Input: part model. Units: mm. Frame: model coordinates. A direction names the side the tool comes from. Round coordinates to 2 decimals unless told otherwise and drop trailing zeros. Loops run counter-clockwise (first coordinate to the right, second up) from the corner with the lowest first, then second, coordinate; pieces in that order, holes last.
(1) Line query: line 1 (X direction, y = 7.25, z = 0); line 2 (Z direction, x = -8, y = 5.5); line 3 (Y direction, x = -20.5, z = -18). Output: solid intervals per line, ascending.
(2) First-contact query: pin 1 Ø0.8 at (y, z) = (4.5, 26) entering from +X; pin 2 Ø0.5 at (x, z) = (-2.5, 30) entering from -Y; pin 3 Ø20.5 at (y, z) = (-0.5, 44.5) entering from +X. Flat tips, straight axial feed; report the tip coordinate or a pass-through.
(3) Cut plane B-B, the plane x = 22. Output: boundary loops of the cut face in (y, z), and give its area (3 significant figures).
(4) Cut plane A-A, the plane z = 0. Output: boundary loops of the cut face in (x, y).
(5) Cut plane D-D, the plane y = -13. Output: boundary loops of the cut face in (x, z), and give its area (3 significant figures).
(6) Cut plane C-C, the plane y = 4. Output: boundary loops of the cut face in (x, z).
(7) Draft query along X for faces 1 (the face through (0, -20, 78)), 2 (the face through (-29.97, 4.93, -1.32)), 3 (the face through (-5, 0, 56)), 4 (the face through (-2.5, 5, -22)). Return one class per face: released by +X, released by -X, zero draft, split by the parting line, or undercut.
(8) Access query for faces 5 (the face through (24.995, 4.93, -0.515)), 6 (the face through (0.07, -2.89, 53.9)), 7 (the face through (0.81, -14.93, 84.31)), 8 (the face through (5, 0, 56)). Directions: +Z, -Z, +X, -X, +Y, -Y. A direction counts if a zero-diameter tool reaches every point of the face in a straight line with its end or side. Return the directions, or none.
from build123d import *

# Parameters (mm, degrees)
SKETCH1_R           = 30
SKETCH1_R_2         = 15
BOSS_EXTRUDE1_DEPTH = 10
BOSS_EXTRUDE2_DEPTH = 5
SKETCH3_R           = 3.75
BOSS_EXTRUDE3_DEPTH = 10
SKETCH5_R           = 2.5
BOSS_EXTRUDE4_DEPTH = 20
BOSS_EXTRUDE4_TAPER = 7


with BuildPart() as part:
    # Sketch1 → Boss-Extrude1 (new body)
    with BuildSketch(Plane(origin=(0, 0, 0), x_dir=(1, 0, 0), z_dir=(0, 1, 0))):
        Circle(SKETCH1_R)
        with BuildLine():
            ThreePointArc((-2.5, -24.874685928), (-25, 0), (-2.5, 24.874685928))
            Line((-2.5, 24.874685928), (-2.5, 19.843134833))
            ThreePointArc((-2.5, 19.843134833), (0, -20), (2.5, 19.843134833))
            Line((2.5, 19.843134833), (2.5, 24.874685928))
            ThreePointArc((2.5, 24.874685928), (25, 0), (2.5, -24.874685928))
            Line((2.5, -24.874685928), (2.5, -26.5))
            ThreePointArc((2.5, -26.5), (2.207106781, -27.207106781), (1.5, -27.5))
            Line((1.5, -27.5), (-1.5, -27.5))
            ThreePointArc((-1.5, -27.5), (-2.207106781, -27.207106781), (-2.5, -26.5))
            Line((-2.5, -26.5), (-2.5, -24.874685928))
        make_face(mode=Mode.SUBTRACT)
        Circle(SKETCH1_R_2, mode=Mode.SUBTRACT)
    extrude(amount=BOSS_EXTRUDE1_DEPTH)

    # Sketch2 → Boss-Extrude2 (add, symmetric)
    with BuildSketch(Plane(origin=(0, 0, 0), x_dir=(0, 0, -1), z_dir=(1, 0, 0))):
        with BuildLine():
            Line((-84.861603584, -10), (-76.4, -10))
            ThreePointArc((-76.4, -10), (-53.579230072, -2.810886638), (-30, 1.25))
            Line((-30, 1.25), (-27.5, 1.25))
            Line((-27.5, 1.25), (-27.5, 8.75))
            Line((-27.5, 8.75), (-30, 8.75))
            ThreePointArc((-30, 8.75), (-58.40777346, 2.778023012), (-85.317259729, -8.109844128))
            ThreePointArc((-85.317259729, -8.109844128), (-85.833754774, -9.234354569), (-84.861603584, -10))
        make_face()
    extrude(amount=BOSS_EXTRUDE2_DEPTH, both=True)

    # Sketch3 → Boss-Extrude3 (add)
    with BuildSketch(Plane(origin=(0, -10, 0), x_dir=(-1, 0, 0), z_dir=(0, -1, 0))):
        with Locations((0, -80.65)):
            Circle(SKETCH3_R)
    extrude(amount=BOSS_EXTRUDE3_DEPTH)

    # Sketch5 → Boss-Extrude4 (add)
    with BuildSketch(Plane(origin=(0, -20, 0), x_dir=(-1, 0, 0), z_dir=(0, -1, 0))):
        with Locations((0, -80.65)):
            Circle(SKETCH5_R)
    extrude(amount=BOSS_EXTRUDE4_DEPTH, taper=BOSS_EXTRUDE4_TAPER)


solid = part.part
Reported:
1. line 1: x = -30 to -25, -20 to -15, 15 to 20, 25 to 30
1. line 2: z = -28.91 to -23.69, -18.33 to -12.69, 12.69 to 18.33, 23.69 to 28.91
1. line 3: y = 0 to 10
2. pin 1: stops at x = 15.64
2. pin 2: stops at y = 0
2. pin 3: stops at x = 5
3. outline: (0, -20.4) - (10, -20.4) - (10, -11.87) - (0, -11.87) - close; (0, 11.87) - (10, 11.87) - (10, 20.4) - (0, 20.4) - close
3. area: 170 mm2
4. outline: (-30, 0) - (-25, 0) - (-25, 10) - (-30, 10) - close; (-20, 0) - (-15, 0) - (-15, 10) - (-20, 10) - close; (15, 0) - (20, 0) - (20, 10) - (15, 10) - close; (25, 0) - (30, 0) - (30, 10) - (25, 10) - close
5. outline: circle Ø7.5 at (0, 80.65)
5. area: 44.2 mm2
6. outline: (-5, 29.58) arc R30 ccw (long way) to (5, 29.58) - (5, 54.2) - (-5, 54.2) - close; hole circle Ø30 at (0, 0); hole (-2.5, -24.87) - (-2.5, -19.84) arc R20 cw (long way) to (2.5, -19.84) - (2.5, -24.87) arc R25 ccw to (2.5, 24.87) - (2.5, 26.5) arc R1 ccw to (1.5, 27.5) - (-1.5, 27.5) arc R1 ccw to (-2.5, 26.5) - (-2.5, 24.87) arc R25 ccw to start
7. face 1: zero draft
7. face 2: split by the parting line
7. face 3: released by -X
7. face 4: undercut
8. face 5: +Y, -Y
8. face 6: +X, -X, -Y
8. face 7: -Y
8. face 8: +Z, +X, +Y, -Y
